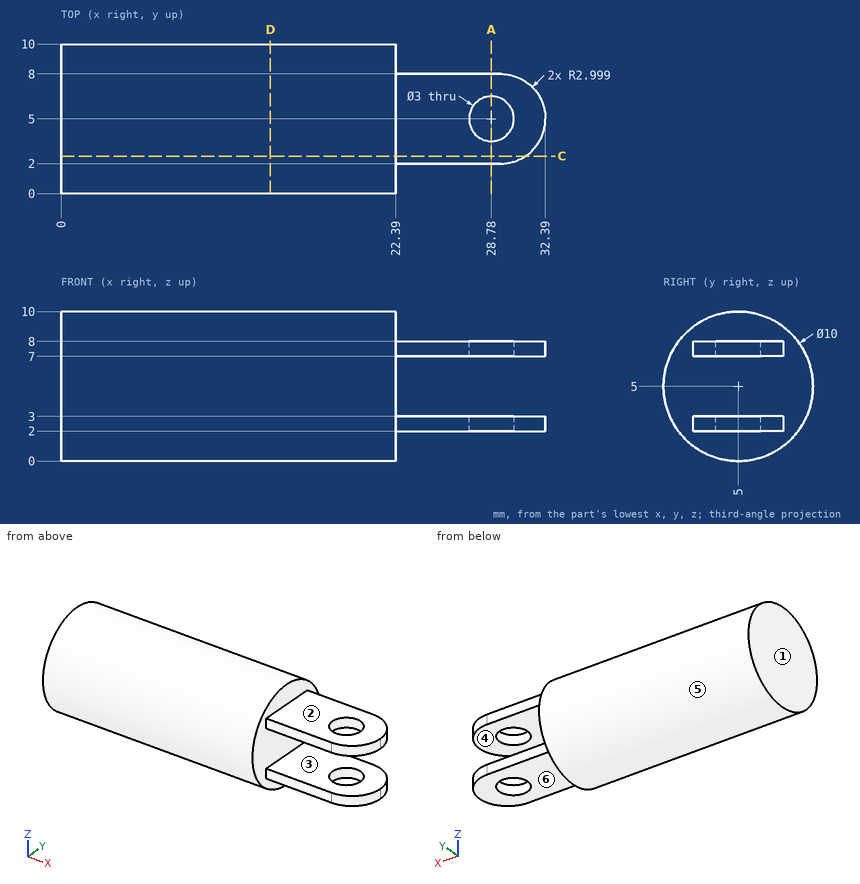
Study the drawing (mm; zero at the part's minimum x, y, z) and answer. A direction names the side the tool comes from. Round coordinates to 2 decimals unless told otherwise and drop trailing zeros. Write each loop counter-clockwise with the first axis right and the second up, starting at its lowest first coordinate (ties: lowest second). Pieces come first, ordered by that corner, then holes. Notation, with made-up numbers: (83.25, -1.75) - (140.25, -1.75) arc R17 cw to (140.25, 10.25) - close; hole circle Ø8 at (65, 35). An arc over 180 degrees is marked (long way). Use CSV: the item, a comma, the result in double quotes.
Q1. A tool of negligible diameter and unlimited length cuts with its end or side. For the marked faces 5 and 6, from which of +Z, -Z, +X, -X, +Y, -Y can it reach the whole face along a straight path? Write none if from no direction.
Values:
face 5,"+X, -X"
face 6,"-Z, +X, +Y, -Y"
Q2. Find section D-D, the plane x = 14. Write down the section's boundary in (y, z).
Values:
outline,"circle Ø10 at (5, 5)"
Q3. Find section C-C, the plane y = 2.5. Write down the section's boundary in (x, z).
Values:
outline,"(0, 0.67) - (22.39, 0.67) - (22.39, 2) - (31.05, 2) - (31.05, 3) - (22.39, 3) - (22.39, 7) - (31.05, 7) - (31.05, 8) - (22.39, 8) - (22.39, 9.33) - (0, 9.33) - close"
Q4. Find section A-A, the plane x = 28.78. Write down the section's boundary in (y, z).
Values:
outline,"(2, 2) - (3.5, 2) - (3.5, 3) - (2, 3) - close; (2, 7) - (3.5, 7) - (3.5, 8) - (2, 8) - close; (6.5, 2) - (8, 2) - (8, 3) - (6.5, 3) - close; (6.5, 7) - (8, 7) - (8, 8) - (6.5, 8) - close"
Q5. Straight lines are drawn through the part: line 1 along Z through (x, y) = (25.5, 3); line 2 along Y through (x, z) = (28.78, 2.4); line 3 along X through (y, z) = (5, 8.25). For each, find the intervals that lie inside material, in ascending order.
Values:
line 1,"z = 2 to 3, 7 to 8"
line 2,"y = 2 to 3.5, 6.5 to 8"
line 3,"x = 0 to 22.39"
Q6. Each of these flat-tipped pins is pushed along its axis until it touches: pin 1 Ø3 at (x, y) = (27, 5) entering from -Z; pin 2 Ø1.5 at (x, z) = (13, 4) entering from +Y; pin 3 Ø4 at (y, z) = (3.5, 7) entering from +X; pin 4 Ø5 at (x, y) = (29, 4.5) entering from +Z. Where does it stop, or does it pass through?
Values:
pin 1,"stops at z = 2"
pin 2,"stops at y = 9.99"
pin 3,"stops at x = 32.39"
pin 4,"stops at z = 8"
Q7. Determine the mould class of the marked faces 1, 2, 3 and 4 for opening direction Z: +Z half, -Z half, draft (parallel to the pull), parting line (faces both ways), or undercut.
Values:
face 1,"draft"
face 2,"+Z half"
face 3,"undercut"
face 4,"undercut"
